Job drawing, mm, ordinate dimensions from the low corner. One solid piece. A direction names the side the tool comes from. Give positions to 0.01 mm unless a question says otherwise; leave off trailing zeros. Order: outer loops, then holes, each group sorted by start corner. A loop starts at its lowest first (then second) coordinate and runs counter-clockwise, first axis right, second up.
Item 1: Band-saw the part on B-B on y = 31.5. Give the cut face in (x, z).
Item 2: Band-saw the part on D-D on x = 4. Give the cut face in (y, z).
Item 3: Band-saw the part on A-A on z = 37.5. Give the cut face in (x, y).
Item 4: Band-saw the part on C-C on z = 29. Give the cut face in (x, y) (1 decimal), plus the area to 3 significant figures.
Item 5: Flat gauge pins, fed straight in: P1, Ø8, axis at x = 52.5, y = 12, coming from the +Z side; P2, Ø6, axis at y = 23.5, z = 44.5, coming from the -X side; P3, Ø6, axis at x = 25, z = 55.5, coming from the +Y side. Where does each tip first touch, or does it go through?
Item 6: Wall check: L1, parallel to Z at x = 46.5, y = 35; L2, parallel to X at y = 29, z = 47 (1 decimal); L3, parallel to Y at x = 26.5, z = 16. Give the ranges that are in metal, low to high.
Item 7: Which spindle directions (+Z, -Z, +X, -X, +Y, -Y) get a long thin tool onto all of the face, cutting with end or side? Do the marked faces 1, 2, 3 and 4. Say none if no direction does.
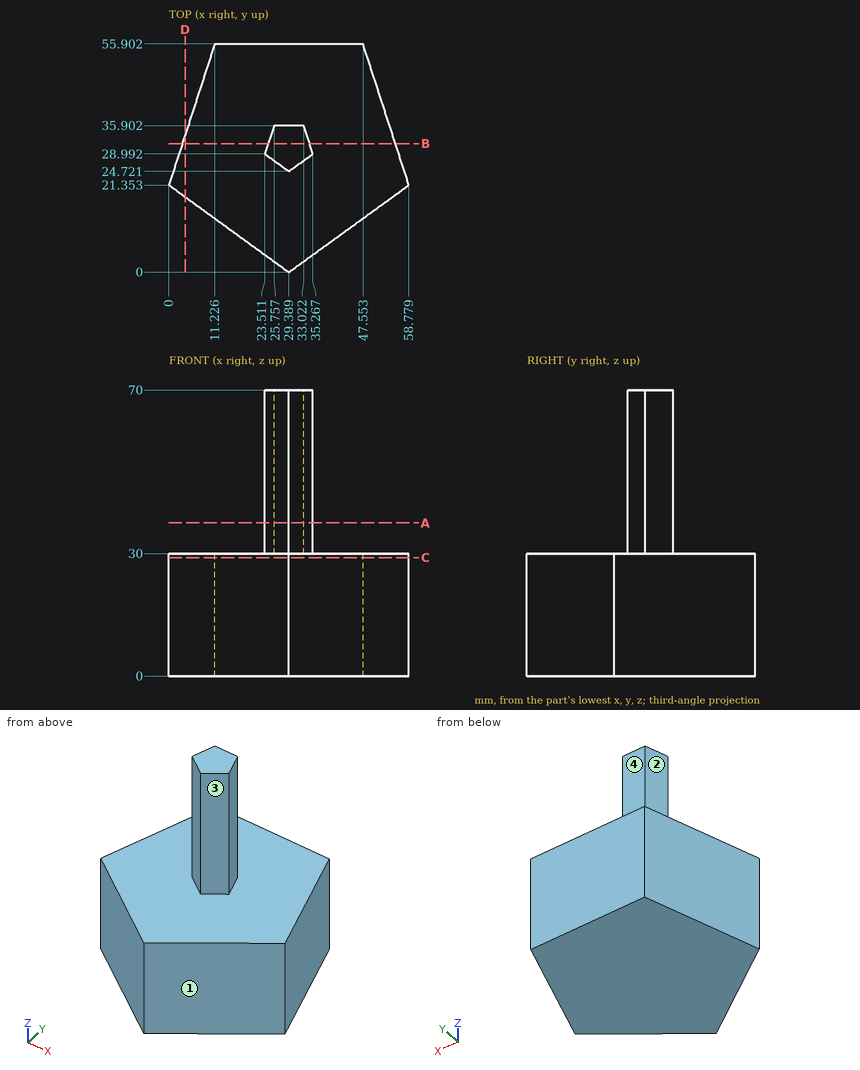
The answers:
1. outline: (3.3, 0) - (55.48, 0) - (55.48, 30) - (34.45, 30) - (34.45, 70) - (24.33, 70) - (24.33, 30) - (3.3, 30) - close
2. outline: (18.45, 0) - (33.66, 0) - (33.66, 30) - (18.45, 30) - close
3. outline: (23.51, 28.99) - (29.39, 24.72) - (35.27, 28.99) - (33.02, 35.9) - (25.76, 35.9) - close
4. outline: (0, 21.4) - (29.4, 0) - (58.8, 21.4) - (47.6, 55.9) - (11.2, 55.9) - close
4. area: 2,270 mm2
5. P1: stops at z = 30
5. P2: stops at x = 26.94
5. P3: stops at y = 35.9
6. L1: z = 0 to 30
6. L2: x = 23.5 to 35.3
6. L3: y = 2.1 to 55.9
7. face 1: +Z, -Z, +X, -Y
7. face 2: +Z, -X, +Y
7. face 3: +Z, +X, -Y
7. face 4: +Z, +X, -X, +Y
